Work out the finished part from the listing and answer in its coordinate system (mm). Face numbers are marked on the shaded views. A direction names the side the tool comes from. Round coordinates to 2 decimals unless told otherwise and drop trailing zeros. Loops run counter-clockwise (first coordinate to the right, second up) from the corner with the lowest first, then second, coordinate; pieces in that order, holes last. Notation, with made-up numbers: (10.25, 62.5) - (19.25, 62.5) arc R24 cw to (19.25, 99.5) - close; hole circle Ø5 at (20, -11.75). An arc over 180 degrees is marked (long way). Answer as CSV lines item,"result". Start each with the question number.
Q1. Each of these flat-tipped pins is pushed along its axis until it touches: pin 1 Ø1 at (y, z) = (10.5, 9.5) entering from +X; pin 2 Ø8 at (y, z) = (-12.5, -2) entering from +X; pin 3 Ø1.5 at (y, z) = (-12, -6.5) entering from +X. Where does it stop, or does it pass through?
Q2. Section A-A on z = 4 is taken. Write down the section's boundary in (x, y), then the cut area to 3 significant figures.
Q3. For the marked faces 1 and 2, determine the directions among +Z, -Z, +X, -X, +Y, -Y from which every point of the face is accessible in a straight line to the end or side of a thin tool.
Q4. Straight lines are drawn through the part: L1, parallel to X at y = -7, z = 5; L2, parallel to X at y = -8, z = 4. For each, find the intervals that lie inside material, in ascending order. Write a range as [from, to].
Q5. Section B-B on y = 12.5 is taken. Write down the section's boundary in (x, z).
```python
from build123d import *

# Parameters (mm, degrees)
SKETCH1_W               = 38.1
SKETCH1_H               = 38.1
BOSS_EXTRUDE1_DEPTH     = 394.2334
CUT_EXTRUDE1_DEPTH      = 397.528039583
CUT_EXTRUDE2_DEPTH      = 397.528039583
CUT_EXTRUDE2_DEPTH_BACK = 397.528039583


with BuildPart() as part:
    # Sketch1 → Boss-Extrude1 (new body)
    with BuildSketch(Plane(origin=(0, 0, 0), x_dir=(0, 0, -1), z_dir=(1, 0, 0))):
        Rectangle(SKETCH1_W, SKETCH1_H)
    extrude(amount=BOSS_EXTRUDE1_DEPTH)

    # Sketch2 → Cut-Extrude1 (cut, through all)
    with BuildSketch(Plane.XY.offset(19.05)):
        Polygon((394.2334, -19.05), (382.468621152, 19.05), (394.2334, 19.05), align=None)
    extrude(amount=-CUT_EXTRUDE1_DEPTH, mode=Mode.SUBTRACT)

    # Sketch3 → Cut-Extrude2 (cut, two sides: drawn at the far end of the back side and taken through both)
    with BuildSketch(Plane.XY.offset(19.05).offset(-CUT_EXTRUDE2_DEPTH_BACK)):
        Polygon((0, 19.05), (0, -5.758314958), (20.522286578, 0.578697196), (14.818591236, 19.05), align=None)
    extrude(amount=CUT_EXTRUDE2_DEPTH + CUT_EXTRUDE2_DEPTH_BACK, mode=Mode.SUBTRACT)


solid = part.part
```
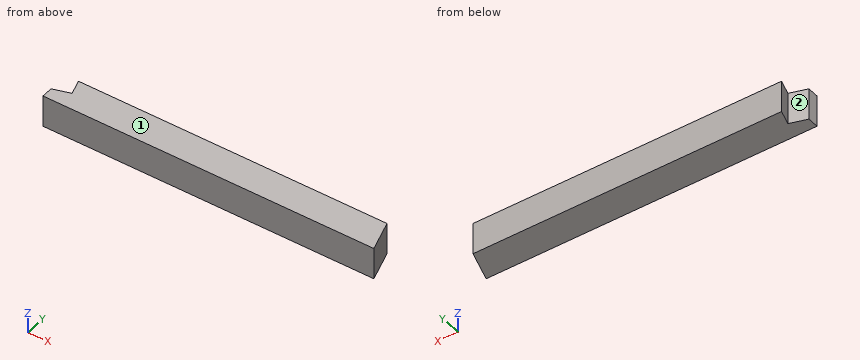
Findings:
1,pin 1,"stops at x = 385.26"
1,pin 2,"stops at x = 393.45"
1,pin 3,"stops at x = 392.29"
2,outline,"(0, -19.05) - (394.23, -19.05) - (382.47, 19.05) - (14.82, 19.05) - (20.52, 0.58) - (0, -5.76) - close"
2,area,"14,400 mm^2"
3,face 1,"+Z, +X, -X, +Y, -Y"
3,face 2,"+Z, -Z, -X"
4,L1,"x = [0, 390.51]"
4,L2,"x = [0, 390.82]"
5,outline,"(16.84, -19.05) - (384.49, -19.05) - (384.49, 19.05) - (16.84, 19.05) - close"
